Input: part model. Units: mm. Frame: model coordinates. Face numbers are marked on the shaded views. A direction names the side the tool comes from. Give positions to 0.01 mm unless a question says otherwise; leave off trailing zeros. Write each loop counter-clockwise with the first axis right and the second up, starting at its lowest first coordinate (ties: lowest second). Pieces come first, ordered by that corner, then holes. Notation, with made-up numbers: (-11.75, 43) - (20.25, 43) arc R17 cw to (20.25, 57) - close; hole circle Ø8 at (-15.5, 47). An arc over 180 degrees is marked (long way). Answer as CSV lines item,"result".
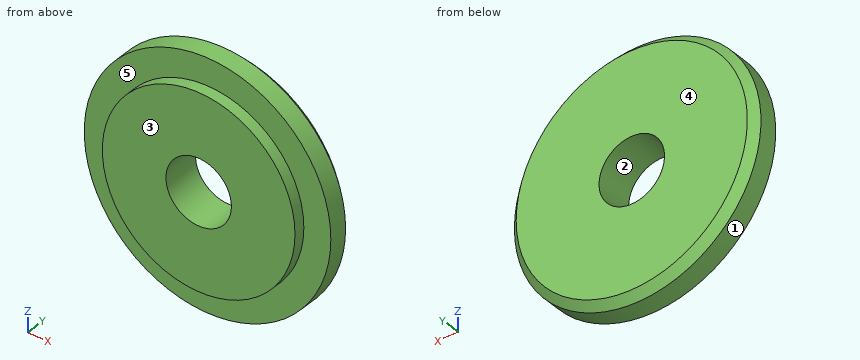
```python
from build123d import *

# Parameters (mm, degrees)
F0_R     = 16
F1_DEPTH = 5
F2_R     = 23.291419
F2_R_2   = 12.5
F3_DEPTH = 1.5
F4_SIZE  = 1
F5_R     = 4.25
F6_DEPTH = 25


with BuildPart() as f1:
    # F0 (on Front) → F1 (new body)
    with BuildSketch(Plane.XZ):
        Circle(F0_R)
    extrude(amount=F1_DEPTH)

    # F2 (on face) → F3 (cut)
    with BuildSketch(Plane.XZ.offset(5)):
        Circle(F2_R)
        Circle(F2_R_2, mode=Mode.SUBTRACT)
    extrude(amount=-F3_DEPTH, mode=Mode.SUBTRACT)

    # F4
    f4_edges = [f1.edges().sort_by_distance(p)[0] for p in [
        (-16, 0, 0),
    ]]
    chamfer(f4_edges, length=F4_SIZE)

    # F5 (on face) → F6 (cut)
    with BuildSketch(Plane.XZ.offset(5)):
        Circle(F5_R)
    extrude(amount=-F6_DEPTH, mode=Mode.SUBTRACT)


solid = f1.part
```
Item 1: Mould query, pull axis X, two halves, no side actions, for the marked faces 1, 2 and 3. Classes: +X half, -X half, draft (parallel to the pull), parting line (faces both ways), or undercut.
The answers:
face 1,"parting line"
face 2,"undercut"
face 3,"draft"
Item 2: Reachability of the marked faces 4 and 5 from +Z, -Z, +X, -X, +Y, -Y: full face, straight path, thin tool, end or side. Return the list, or none.
The answers:
face 4,"+Z, -Z, +X, -X, +Y"
face 5,"-Y"
Item 3: Contact query for a flat-ended pin moving along its axis: pin 1 (3 mm diameter, centred on y = -3, z = 5, fed in from -X). Output: stop coordinate, or through.
The answers:
pin 1,"x = -15.61"
Item 4: Ray query, line 1 (Z direction, x = 0, y = -3.3); line 2 (Z direction, x = 0, y = -3.95); line 3 (Y direction, x = -9.5, z = 11.5). Return the intervals inside material, ascending. Write a range as from..to.
The answers:
line 1,"-16..-4.25, 4.25..16"
line 2,"-12.5..-4.25, 4.25..12.5"
line 3,"-3.5..0"
Item 5: Cut plane B-B on x = 0. Return the cut outline in (y, z).
The answers:
outline,"(-5, -12.5) - (-3.5, -12.5) - (-3.5, -16) - (-1, -16) - (0, -15) - (0, -4.25) - (-5, -4.25) - close; (-5, 4.25) - (0, 4.25) - (0, 15) - (-1, 16) - (-3.5, 16) - (-3.5, 12.5) - (-5, 12.5) - close"
Item 6: Cut plane A-A on z = 0. Return the cut outline in (x, y), plus the area to 3 significant figures.
The answers:
outline,"(-16, -3.5) - (-12.5, -3.5) - (-12.5, -5) - (-4.25, -5) - (-4.25, 0) - (-15, 0) - (-16, -1) - close; (4.25, -5) - (12.5, -5) - (12.5, -3.5) - (16, -3.5) - (16, -1) - (15, 0) - (4.25, 0) - close"
area,"106 mm²"
